Geometry: final body of the model. Coordinates: model frame, mm. A direction names the side the tool comes from. Give positions to 0.01 mm unless a question says otherwise; leave off trailing zeros. Order: outer loops, then holes, each group sorted by start corner. A loop starts at its lowest first (then second) coordinate and runs counter-clockwise, first axis right, second up. Notation, with made-up numbers: (44.25, 74) -> (64.25, 74) arc R30 cw to (64.25, 107) -> close; hole circle Ø9 at (30, 18.5). An arc over 180 degrees is marked (long way). One line per question, with ' | ' between items.
from build123d import *

# Parameters (mm, degrees)
F0_W     = 1.4
F0_H     = 1.4
F0_W_2   = 1.65
F0_H_2   = 1.65
F1_DEPTH = 2


with BuildPart() as f1:
    # F0 (on Top) → F1 (new body)
    with BuildSketch(Plane.XY):
        with BuildLine():
            ThreePointArc((-21.2961866601, -12.2818885401), (-21.155367688, -11.7070138204), (-20.9225061022, -11.1628755952))
            ThreePointArc((-20.9225061022, -11.1628755952), (-21.5623124485, -11.234937617), (-22.186206323, -11.3940021608))
            ThreePointArc((-22.186206323, -11.3940021608), (-22.3437732086, -12.0182759568), (-22.4142996364, -12.6582533929))
            ThreePointArc((-22.4142996364, -12.6582533929), (-21.8707217917, -12.4240866724), (-21.2961866601, -12.2818885401))
        make_face()
        with BuildLine():
            ThreePointArc((-22.186206323, -11.3940021608), (-21.5623124485, -11.234937617), (-20.9225061022, -11.1628755952))
            ThreePointArc((-20.9225061022, -11.1628755952), (-17.7315900511, -9.2404582472), (-14.5403036541, -11.1622607443))
            ThreePointArc((-14.5403036541, -11.1622607443), (-13.9013713953, -11.2321194541), (-13.278004152, -11.3887334725))
            ThreePointArc((-13.278004152, -11.3887334725), (-17.7340143596, -8.1634590502), (-22.186206323, -11.3940021608))
        make_face()
        with BuildLine():
            ThreePointArc((-22.4142996364, -12.6582533929), (-22.3437732086, -12.0182759568), (-22.186206323, -11.3940021608))
            ThreePointArc((-22.186206323, -11.3940021608), (-25.4060635692, -15.8454582305), (-22.186206323, -20.2969143001))
            ThreePointArc((-22.186206323, -20.2969143001), (-22.3437732086, -19.6726405041), (-22.4142996364, -19.032663068))
            ThreePointArc((-22.4142996364, -19.032663068), (-24.3290635692, -15.8454582305), (-22.4142996364, -12.6582533929))
        make_face()
        with BuildLine():
            ThreePointArc((-13.278004152, -11.3887334725), (-13.9013713953, -11.2321194541), (-14.5403036541, -11.1622607443))
            ThreePointArc((-14.5403036541, -11.1622607443), (-14.3076050054, -11.7055530453), (-14.1666742594, -12.2795336289))
            ThreePointArc((-14.1666742594, -12.2795336289), (-13.5923579293, -12.4190898486), (-13.0485100994, -12.6504871765))
            ThreePointArc((-13.0485100994, -12.6504871765), (-13.1198982272, -12.011723992), (-13.278004152, -11.3887334725))
        make_face()
        with BuildLine():
            ThreePointArc((-22.4142996364, -19.032663068), (-22.3437732086, -19.6726405041), (-22.186206323, -20.2969143001))
            ThreePointArc((-22.186206323, -20.2969143001), (-21.5623124485, -20.455978844), (-20.9225061022, -20.5280408657))
            ThreePointArc((-20.9225061022, -20.5280408657), (-21.155367688, -19.9839026405), (-21.2961866601, -19.4090279208))
            ThreePointArc((-21.2961866601, -19.4090279208), (-21.8707217917, -19.2668297885), (-22.4142996364, -19.032663068))
        make_face()
        with BuildLine():
            ThreePointArc((-20.9225061022, -20.5280408657), (-21.5623124485, -20.455978844), (-22.186206323, -20.2969143001))
            ThreePointArc((-22.186206323, -20.2969143001), (-17.7340143596, -23.5274574107), (-13.278004152, -20.3021829884))
            ThreePointArc((-13.278004152, -20.3021829884), (-13.9013713953, -20.4587970068), (-14.5403036541, -20.5286557166))
            ThreePointArc((-14.5403036541, -20.5286557166), (-17.7315900511, -22.4504582137), (-20.9225061022, -20.5280408657))
        make_face()
        with BuildLine():
            ThreePointArc((-13.278004152, -20.3021829884), (-10.0420635692, -15.8454582305), (-13.278004152, -11.3887334725))
            ThreePointArc((-13.278004152, -11.3887334725), (-13.1198982272, -12.011723992), (-13.0485100994, -12.6504871765))
            ThreePointArc((-13.0485100994, -12.6504871765), (-11.1190635692, -15.8454582305), (-13.0485100994, -19.0404292844))
            ThreePointArc((-13.0485100994, -19.0404292844), (-13.1198982272, -19.6791924689), (-13.278004152, -20.3021829884))
        make_face()
        with BuildLine():
            ThreePointArc((-14.5403036541, -20.5286557166), (-13.9013713953, -20.4587970068), (-13.278004152, -20.3021829884))
            ThreePointArc((-13.278004152, -20.3021829884), (-13.1198982272, -19.6791924689), (-13.0485100994, -19.0404292844))
            ThreePointArc((-13.0485100994, -19.0404292844), (-13.5923579293, -19.2718266123), (-14.1666742594, -19.4113828321))
            ThreePointArc((-14.1666742594, -19.4113828321), (-14.3076050054, -19.9853634156), (-14.5403036541, -20.5286557166))
        make_face()
        with BuildLine():
            ThreePointArc((-21.3412422696, -12.8504582305), (-21.3299607394, -12.565282188), (-21.2961866601, -12.2818885401))
            ThreePointArc((-21.2961866601, -12.2818885401), (-21.8707217917, -12.4240866724), (-22.4142996364, -12.6582533929))
            ThreePointArc((-22.4142996364, -12.6582533929), (-22.4172565076, -12.7543355953), (-22.4182422696, -12.8504582305))
            Line((-22.4182422696, -12.8504582305), (-22.4182422696, -15.0204582305))
            Line((-22.4182422696, -15.0204582305), (-19.9490635692, -15.0204582305))
            Line((-19.9490635692, -15.0204582305), (-19.9490635692, -13.6204582305))
            Line((-19.9490635692, -13.6204582305), (-21.3412422696, -13.6204582305))
            Line((-21.3412422696, -13.6204582305), (-21.3412422696, -12.8504582305))
        make_face()
        with Locations((-19.2490635692, -14.3204582305)):
            Rectangle(F0_W, F0_H)
        with BuildLine():
            Line((-18.5490635692, -11.1584582305), (-20.7190635692, -11.1584582305))
            ThreePointArc((-20.7190635692, -11.1584582305), (-20.8208088115, -11.1595627018), (-20.9225061022, -11.1628755952))
            ThreePointArc((-20.9225061022, -11.1628755952), (-21.155367688, -11.7070138204), (-21.2961866601, -12.2818885401))
            ThreePointArc((-21.2961866601, -12.2818885401), (-21.0085574533, -12.2470845296), (-20.7190635692, -12.2354582305))
            Line((-20.7190635692, -12.2354582305), (-19.9490635692, -12.2354582305))
            Line((-19.9490635692, -12.2354582305), (-19.9490635692, -13.6204582305))
            Line((-19.9490635692, -13.6204582305), (-18.5490635692, -13.6204582305))
            Line((-18.5490635692, -13.6204582305), (-18.5490635692, -11.1584582305))
        make_face()
        with Locations((-17.7240635692, -14.3204582305)):
            Rectangle(F0_W_2, F0_H)
        with Locations((-16.1990635692, -14.3204582305)):
            Rectangle(F0_W, F0_H)
        with BuildLine():
            ThreePointArc((-13.0485100994, -12.6504871765), (-13.5923579293, -12.4190898486), (-14.1666742594, -12.2795336289))
            ThreePointArc((-14.1666742594, -12.2795336289), (-14.1326181911, -12.5640935301), (-14.1212422696, -12.8504582305))
            Line((-14.1212422696, -12.8504582305), (-14.1212422696, -13.6204582305))
            Line((-14.1212422696, -13.6204582305), (-15.4990635692, -13.6204582305))
            Line((-15.4990635692, -13.6204582305), (-15.4990635692, -15.0204582305))
            Line((-15.4990635692, -15.0204582305), (-13.0442422696, -15.0204582305))
            Line((-13.0442422696, -15.0204582305), (-13.0442422696, -12.8504582305))
            ThreePointArc((-13.0442422696, -12.8504582305), (-13.0453093485, -12.7504499348), (-13.0485100994, -12.6504871765))
        make_face()
        with BuildLine():
            ThreePointArc((-14.1666742594, -12.2795336289), (-14.3076050054, -11.7055530453), (-14.5403036541, -11.1622607443))
            ThreePointArc((-14.5403036541, -11.1622607443), (-14.6346644635, -11.1594089553), (-14.7290635692, -11.1584582305))
            Line((-14.7290635692, -11.1584582305), (-16.8990635692, -11.1584582305))
            Line((-16.8990635692, -11.1584582305), (-16.8990635692, -13.6204582305))
            Line((-16.8990635692, -13.6204582305), (-15.4990635692, -13.6204582305))
            Line((-15.4990635692, -13.6204582305), (-15.4990635692, -12.2354582305))
            Line((-15.4990635692, -12.2354582305), (-14.7290635692, -12.2354582305))
            ThreePointArc((-14.7290635692, -12.2354582305), (-14.4470066704, -12.2464939481), (-14.1666742594, -12.2795336289))
        make_face()
        with BuildLine():
            ThreePointArc((-14.7290635692, -20.5324582305), (-14.6346644635, -20.5315075056), (-14.5403036541, -20.5286557166))
            ThreePointArc((-14.5403036541, -20.5286557166), (-14.3076050054, -19.9853634156), (-14.1666742594, -19.4113828321))
            ThreePointArc((-14.1666742594, -19.4113828321), (-14.4470066704, -19.4444225128), (-14.7290635692, -19.4554582305))
            Line((-14.7290635692, -19.4554582305), (-15.4990635692, -19.4554582305))
            Line((-15.4990635692, -19.4554582305), (-15.4990635692, -18.0704582305))
            Line((-15.4990635692, -18.0704582305), (-16.8990635692, -18.0704582305))
            Line((-16.8990635692, -18.0704582305), (-16.8990635692, -20.5324582305))
            Line((-16.8990635692, -20.5324582305), (-14.7290635692, -20.5324582305))
        make_face()
        with BuildLine():
            ThreePointArc((-14.1666742594, -19.4113828321), (-13.5923579293, -19.2718266123), (-13.0485100994, -19.0404292844))
            ThreePointArc((-13.0485100994, -19.0404292844), (-13.0453093485, -18.9404665261), (-13.0442422696, -18.8404582305))
            Line((-13.0442422696, -18.8404582305), (-13.0442422696, -16.6704582305))
            Line((-13.0442422696, -16.6704582305), (-15.4990635692, -16.6704582305))
            Line((-15.4990635692, -16.6704582305), (-15.4990635692, -18.0704582305))
            Line((-15.4990635692, -18.0704582305), (-14.1212422696, -18.0704582305))
            Line((-14.1212422696, -18.0704582305), (-14.1212422696, -18.8404582305))
            ThreePointArc((-14.1212422696, -18.8404582305), (-14.1326181911, -19.1268229308), (-14.1666742594, -19.4113828321))
        make_face()
        with Locations((-16.1990635692, -17.3704582305)):
            Rectangle(F0_W, F0_H)
        with Locations((-16.1990635692, -15.8454582305)):
            Rectangle(F0_W, F0_H_2)
        with Locations((-19.2490635692, -17.3704582305)):
            Rectangle(F0_W, F0_H)
        with Locations((-19.2490635692, -15.8454582305)):
            Rectangle(F0_W, F0_H_2)
        with Locations((-17.7240635692, -17.3704582305)):
            Rectangle(F0_W_2, F0_H)
        with BuildLine():
            ThreePointArc((-21.2961866601, -19.4090279208), (-21.155367688, -19.9839026405), (-20.9225061022, -20.5280408657))
            ThreePointArc((-20.9225061022, -20.5280408657), (-20.8208088115, -20.5313537591), (-20.7190635692, -20.5324582305))
            Line((-20.7190635692, -20.5324582305), (-18.5490635692, -20.5324582305))
            Line((-18.5490635692, -20.5324582305), (-18.5490635692, -18.0704582305))
            Line((-18.5490635692, -18.0704582305), (-19.9490635692, -18.0704582305))
            Line((-19.9490635692, -18.0704582305), (-19.9490635692, -19.4554582305))
            Line((-19.9490635692, -19.4554582305), (-20.7190635692, -19.4554582305))
            ThreePointArc((-20.7190635692, -19.4554582305), (-21.0085574533, -19.4438319313), (-21.2961866601, -19.4090279208))
        make_face()
        with BuildLine():
            ThreePointArc((-22.4182422696, -18.8404582305), (-22.4172565076, -18.9365808656), (-22.4142996364, -19.032663068))
            ThreePointArc((-22.4142996364, -19.032663068), (-21.8707217917, -19.2668297885), (-21.2961866601, -19.4090279208))
            ThreePointArc((-21.2961866601, -19.4090279208), (-21.3299607394, -19.1256342729), (-21.3412422696, -18.8404582305))
            Line((-21.3412422696, -18.8404582305), (-21.3412422696, -18.0704582305))
            Line((-21.3412422696, -18.0704582305), (-19.9490635692, -18.0704582305))
            Line((-19.9490635692, -18.0704582305), (-19.9490635692, -16.6704582305))
            Line((-19.9490635692, -16.6704582305), (-22.4182422696, -16.6704582305))
            Line((-22.4182422696, -16.6704582305), (-22.4182422696, -18.8404582305))
        make_face()
    extrude(amount=F1_DEPTH)


solid = f1.part
1) Section B-B on x = -21.75. Return loops of the section in (y, z).
Check result:
outline: (-21.25, 0) -> (-16.67, 0) -> (-16.67, 2) -> (-21.25, 2) -> close; (-15.02, 0) -> (-10.44, 0) -> (-10.44, 2) -> (-15.02, 2) -> close
2) Pull-direction query (Y, two-part tool) for faces 1 (the cylindrical face through (-17.652, -8.164, 0.986)), 2 (the flat face through (-19.949, -19, 1)), 3 (the cylindrical face through (-25.405, -15.763, 0.986)), 4 (the flat face through (-22.418, -14, 1)); classes: +Y half, -Y half, draft (parallel to the pull), parting line (faces both ways), or undercut.
Check result:
face 1: +Y half | face 2: undercut | face 3: parting line | face 4: undercut
3) Section C-C on y = -15.5. Return loops of the section in (x, z), plus the area to 3 significant figures.
Check result:
outline: (-25.39, 0) -> (-24.31, 0) -> (-24.31, 2) -> (-25.39, 2) -> close; (-19.95, 0) -> (-18.55, 0) -> (-18.55, 2) -> (-19.95, 2) -> close; (-16.9, 0) -> (-15.5, 0) -> (-15.5, 2) -> (-16.9, 2) -> close; (-11.14, 0) -> (-10.05, 0) -> (-10.05, 2) -> (-11.14, 2) -> close | area: 9.92 mm^2
4) Material intervals for probe 1 along X at (y, z) = (-16.25, 1.7); probe 2 along Y at (x, z) = (-17.75, 1.4); probe 3 along X at (y, z) = (-18.25, 1.3), sorted ascending. Write a range as from..to.
Check result:
probe 1: x = -25.39..-24.31, -19.95..-18.55, -16.9..-15.5, -11.14..-10.06 | probe 2: y = -23.53..-22.45, -18.07..-16.67, -15.02..-13.62, -9.24..-8.16 | probe 3: x = -24.74..-23.41, -22.42..-21.34, -19.95..-18.55, -16.9..-15.5, -14.12..-13.04, -12.04..-10.71
5) Set-up query: faces 5 (the flat face through (-18.549, -12, 1)), 6 (the flat face through (-19.5, -15.7, 0)). Return all of +Z, -Z, +X, -X, +Y, -Y with unobstructed straight access to the full face (end or side cutting, diameter ignored); none if empty.
Check result:
face 5: +Z, -Z | face 6: -Z, +X, -X, +Y, -Y
6) Section A-A on y = -20.75. Return loops of the section in (x, z).
Check result:
outline: (-22.01, 0) -> (-20.79, 0) -> (-20.79, 2) -> (-22.01, 2) -> close; (-14.67, 0) -> (-13.45, 0) -> (-13.45, 2) -> (-14.67, 2) -> close
7) Contact query for flat-ended pins moving along their axis: pin 1 Ø1 at (y, z) = (-14.5, 0) entering from +X; pin 2 Ø0.7 at (y, z) = (-19, 1) entering from +X; pin 3 Ø0.6 at (y, z) = (-19, 0.5) entering from -X. Output: stop coordinate, or through.
Check result:
pin 1: stops at x = -10.12 | pin 2: stops at x = -10.97 | pin 3: stops at x = -24.44
8) Section D-D on x = -16.5. Return loops of the section in (y, z).
Check result:
outline: (-23.36, 0) -> (-22.23, 0) -> (-22.23, 2) -> (-23.36, 2) -> close; (-20.53, 0) -> (-11.16, 0) -> (-11.16, 2) -> (-20.53, 2) -> close; (-9.46, 0) -> (-8.33, 0) -> (-8.33, 2) -> (-9.46, 2) -> close
